The model under review builds one solid part; all positions refer to its coordinate system, in mm. Face numbers are marked on the shaded views. A direction names the side the tool comes from. Give positions to 0.01 mm unless a question says otherwise; leave off trailing zeros. Order: outer loops, then holes, each group sorted by start corner. A loop starts at its lowest first (then second) coordinate and runs counter-clockwise, first axis right, second up. Notation, with made-up numbers: (19.5, 25) - (66.5, 25) arc R31 ccw to (66.5, 59) - close; hole circle Ø7 at (-2.5, 63). An arc over 180 degrees is marked (long way). Write item = value, one per line. Start each with the question number.
1. For P1, Ø0.5, axis at x = 3.5, y = 11, coming from the -Z side; P2, Ø0.5, axis at x = 58.5, z = 8.5, coming from the -Y side; P3, Ø9, axis at y = 4, z = -9.5, coming from the -X side, all flat-tipped, find the tip position at first contact; note any pin that passes through.
2. Mouldability with a two-part tool opening along X and no side actions: class the marked faces 4, 5, 6 and 7 as pulls with the +X half, pulls with the -X half, needs draft (parallel to the pull), parting line crosses it, or undercut.
3. Wall thickness on probe 1 along X at (y, z) = (10.55, 18); probe 2 along X at (y, z) = (12.05, -18); probe 3 along X at (y, z) = (8.75, -34): over which ranges is each line inside the solid? List them lowest first.
4. Machinability: for the marked faces 1, 2 and 3, which of the approach directions +Z, -Z, +X, -X, +Y, -Y give a long, thin tool a straight path to every point of the face, cutting with its end or side? Answer none if there is none.
5. We need section C-C, the plane y = 0.75. Give the boundary of the cut face in (x, z), and give its area (3 significant figures).
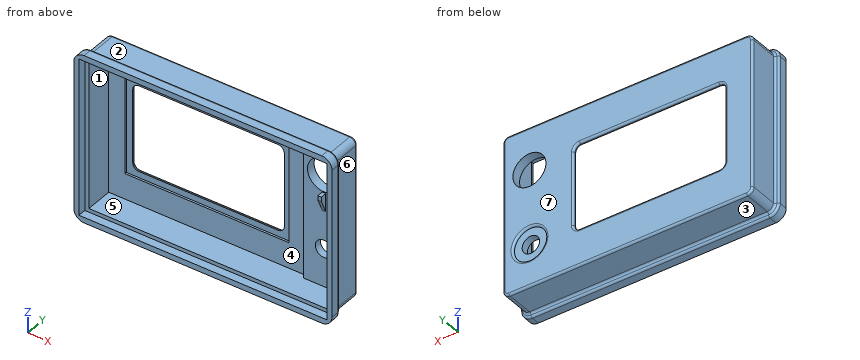
from build123d import *

# Parameters (mm, degrees)
SKETCH1_W                = 122
SKETCH1_H                = 78
SKETCH1_W_2              = 117
SKETCH1_H_2              = 73
BOSS_EXTRUDE1_DEPTH      = 16
SKETCH2_W                = 122
SKETCH2_H                = 78
SKETCH2_W_2              = 74
SKETCH2_H_2              = 42
BOSS_EXTRUDE2_DEPTH      = 2.5
SKETCH3_W                = 80
SKETCH3_H                = 48
CUT_EXTRUDE1_DEPTH       = 1
FILLET1_R                = 3
SKETCH4_R                = 4.25
SKETCH4_R_2              = 8.05
CUT_EXTRUDE2_DEPTH       = 84.00150601
SKETCH5_W                = 20.5
SKETCH5_H                = 73
SKETCH5_R                = 4.25
SKETCH5_R_2              = 8.05
BOSS_EXTRUDE3_DEPTH      = 2
SKETCH6_R                = 8
CUT_EXTRUDE3_DEPTH       = 1
FILLET2_R                = 3
SKETCH7_W                = 1.713480086
SKETCH7_H                = 2
BOSS_EXTRUDE4_DEPTH      = 3
BOSS_EXTRUDE5_DEPTH      = 1.713480086
FILLET3_R                = 1
FILLET4_R                = 1
FILLET5_R                = 1
BOSS_EXTRUDE6_DEPTH      = 4
BOSS_EXTRUDE6_DEPTH_BACK = 1
SKETCH10_W               = 121
SKETCH10_H               = 76.6
CUT_EXTRUDE4_DEPTH       = 86.669422783
FILLET10_R               = 1


with BuildPart() as part:
    # Sketch1 → Boss-Extrude1 (new body)
    with BuildSketch(Plane(origin=(0, -3, 0), x_dir=(1, 0, 0), z_dir=(0, 1, 0))):
        with Locations((10.5, 0)):
            Rectangle(SKETCH1_W, SKETCH1_H)
        with Locations((10.5, 0)):
            Rectangle(SKETCH1_W_2, SKETCH1_H_2, mode=Mode.SUBTRACT)
    extrude(amount=BOSS_EXTRUDE1_DEPTH)

    # Sketch2 → Boss-Extrude2 (add)
    with BuildSketch(Plane(origin=(0, 13, 0), x_dir=(1, 0, 0), z_dir=(0, 1, 0))):
        with Locations((10.5, 0)):
            Rectangle(SKETCH2_W, SKETCH2_H)
        Rectangle(SKETCH2_W_2, SKETCH2_H_2, mode=Mode.SUBTRACT)
    extrude(amount=-BOSS_EXTRUDE2_DEPTH)

    # Sketch3 → Cut-Extrude1 (cut)
    with BuildSketch(Plane.XZ.offset(-10.5)):
        Rectangle(SKETCH3_W, SKETCH3_H)
    extrude(amount=-CUT_EXTRUDE1_DEPTH, mode=Mode.SUBTRACT)

    # Fillet1
    fillet1_edges = [part.edges().sort_by_distance(p)[0] for p in [
        (-50.5, 5, -39),
        (71.5, 5, -39),
        (71.5, 5, 39),
        (-50.5, 5, 39),
    ]]
    fillet(fillet1_edges, radius=FILLET1_R)

    # Sketch4 → Cut-Extrude2 (cut, through all)
    with BuildSketch(Plane(origin=(0, 13, 0), x_dir=(1, 0, 0), z_dir=(0, 1, 0))):
        with Locations(Location((58.5, 18, 0), (0, 0, 270))):
            Circle(SKETCH4_R)
        with Locations(Location((58.5, -18, 0), (0, 0, 270))):
            Circle(SKETCH4_R_2)
    extrude(amount=-CUT_EXTRUDE2_DEPTH, mode=Mode.SUBTRACT)

    # Sketch5 → Boss-Extrude3 (add)
    with BuildSketch(Plane.XZ.offset(-10.5)):
        with Locations((58.75, 0)):
            Rectangle(SKETCH5_W, SKETCH5_H)
        with Locations(Location((58.5, -18, 0), (0, 0, 90))):
            Circle(SKETCH5_R, mode=Mode.SUBTRACT)
        with Locations(Location((58.5, 18, 0), (0, 0, 90))):
            Circle(SKETCH5_R_2, mode=Mode.SUBTRACT)
    extrude(amount=BOSS_EXTRUDE3_DEPTH)

    # Sketch6 → Cut-Extrude3 (cut)
    with BuildSketch(Plane(origin=(0, 13, 0), x_dir=(1, 0, 0), z_dir=(0, 1, 0))):
        with Locations(Location((58.5, 18, 0), (0, 0, 270))):
            Circle(SKETCH6_R)
    extrude(amount=-CUT_EXTRUDE3_DEPTH, mode=Mode.SUBTRACT)

    # Fillet2
    fillet2_edges = [part.edges().sort_by_distance(p)[0] for p in [
        (37, 12.25, 21),
        (-37, 12.25, 21),
        (37, 12.25, -21),
        (-37, 12.25, -21),
    ]]
    fillet(fillet2_edges, radius=FILLET2_R)

    # Sketch7 → Boss-Extrude4 (add)
    with BuildSketch(Plane.XZ.offset(-8.5)):
        with Locations((58.5, 8.5)):
            Rectangle(SKETCH7_W, SKETCH7_H)
    extrude(amount=BOSS_EXTRUDE4_DEPTH)

    # Sketch8 → Boss-Extrude5 (add)
    with BuildSketch(Plane.ZY.offset(-57.643259957)):
        Polygon((7.5, 5.5), (0.486710099, 8.5), (7.5, 8.5), align=None)
    extrude(amount=-BOSS_EXTRUDE5_DEPTH)

    # Fillet3
    fillet3_edges = [part.edges().sort_by_distance(p)[0] for p in [
        (-50.5, 13, 0),
        (10.5, 13, -39),
        (10.5, 13, 39),
        (71.5, 13, 0),
        (70.621320344, 13, 38.121320344),
        (70.621320344, 13, -38.121320344),
        (-49.621320344, 13, 38.121320344),
        (-49.621320344, 13, -38.121320344),
    ]]
    fillet(fillet3_edges, radius=FILLET3_R)

    # Fillet4
    fillet4_edges = [part.edges().sort_by_distance(p)[0] for p in [
        (37, 13, 0),
        (0, 13, 21),
        (-37, 13, 0),
        (0, 13, -21),
        (36.121320344, 13, 20.121320344),
        (-36.121320344, 13, 20.121320344),
        (-36.121320344, 13, -20.121320344),
        (36.121320344, 13, -20.121320344),
    ]]
    fillet(fillet4_edges, radius=FILLET4_R)

    # Fillet5
    fillet5_edges = [part.edges().sort_by_distance(p)[0] for p in [
        (58.5, 13, -26),
    ]]
    fillet(fillet5_edges, radius=FILLET5_R - 0.0001)  # a hair under: the kernel refuses the full size

    # Sketch9 → Boss-Extrude6 (add, two sides: drawn at the far end of the back side and taken through both)
    with BuildSketch(Plane.XZ.offset(3).offset(-BOSS_EXTRUDE6_DEPTH_BACK)):
        with BuildLine():
            Line((-52.5, -36), (-52.5, 36))
            ThreePointArc((-52.5, 36), (-51.035533906, 39.535533906), (-47.5, 41))
            Line((-47.5, 41), (68.5, 41))
            ThreePointArc((68.5, 41), (72.035533906, 39.535533906), (73.5, 36))
            Line((73.5, 36), (73.5, -36))
            ThreePointArc((73.5, -36), (72.035533906, -39.535533906), (68.5, -41))
            Line((68.5, -41), (-47.5, -41))
            ThreePointArc((-47.5, -41), (-51.035533906, -39.535533906), (-52.5, -36))
        make_face()
        with BuildLine():
            Line((-48, 38.3), (69, 38.3))
            ThreePointArc((69, 38.3), (70.414213562, 37.714213562), (71, 36.3))
            Line((71, 36.3), (71, -36.3))
            ThreePointArc((71, -36.3), (70.414213562, -37.714213562), (69, -38.3))
            Line((69, -38.3), (-48, -38.3))
            ThreePointArc((-48, -38.3), (-49.414213562, -37.714213562), (-50, -36.3))
            Line((-50, -36.3), (-50, 36.3))
            ThreePointArc((-50, 36.3), (-49.414213562, 37.714213562), (-48, 38.3))
        make_face(mode=Mode.SUBTRACT)
    extrude(amount=BOSS_EXTRUDE6_DEPTH + BOSS_EXTRUDE6_DEPTH_BACK)

    # Sketch10 → Cut-Extrude4 (cut, through all)
    with BuildSketch(Plane.XZ.offset(3)):
        with Locations((10.5, 0)):
            Rectangle(SKETCH10_W, SKETCH10_H)
    extrude(amount=CUT_EXTRUDE4_DEPTH, mode=Mode.SUBTRACT)

    # Fillet10
    fillet10_edges = [part.edges().sort_by_distance(p)[0] for p in [
        (70.621320344, -2, 38.121320344),
        (-49.621320344, -2, -38.121320344),
        (-49.621320344, -2, 38.121320344),
        (70.621320344, -2, -38.121320344),
        (-51.035533906, -2, 39.535533906),
        (10.5, -2, 41),
        (72.035533906, -2, 39.535533906),
        (73.5, -2, 0),
        (72.035533906, -2, -39.535533906),
        (10.5, -2, -41),
        (-51.035533906, -2, -39.535533906),
        (-52.5, -2, 0),
        (10.5, -2, -39),
        (71.5, -2, 0),
        (10.5, -2, 39),
        (-50.5, -2, 0),
    ]]
    fillet(fillet10_edges, radius=FILLET10_R - 0.0001)  # a hair under: the kernel refuses the full size


solid = part.part
Model answer:
q1.P1 = -39
q1.P2 = 5.5
q1.P3 = -50.5
q2.face_4 = undercut
q2.face_5 = undercut
q2.face_6 = pulls with the +X half
q2.face_7 = needs draft
q3.probe_1 = -50.5 to -40, 40 to 50.45, 66.55 to 71.5
q3.probe_2 = -50.5 to -37, 37 to 50.5, 66.5 to 71.5
q3.probe_3 = -50.5 to -48, 48.5 to 71.5
q4.face_1 = -Y
q4.face_2 = +Z, +X, -X, +Y
q4.face_3 = -Z, +X, -X, +Y
q5.outline = (-50.5, -36) arc R3 ccw to (-47.5, -39) - (68.5, -39) arc R3 ccw to (71.5, -36) - (71.5, 36) arc R3 ccw to (68.5, 39) - (-47.5, 39) arc R3 ccw to (-50.5, 36) - close; hole (-48, -36.5) - (69, -36.5) - (69, 36.5) - (-48, 36.5) - close
q5.area = 967 mm2
